from build123d import *

# Parameters (mm, degrees)
F1_DEPTH = 12.5
F2_W     = 25
F2_H     = 34
F3_DEPTH = 2.5
F4_W     = 25
F4_H     = 2
F5_DEPTH = 30
F6_W     = 2
F6_H     = 25
F7_DEPTH = 20
F8_W     = 32.5
F8_H     = 10
F9_DEPTH = 2


with BuildPart() as f1:
    # F0 (on Front) → F1 (new body, symmetric)
    with BuildSketch(Plane.XZ):
        Polygon((9.5, -9.5), (9.5, 9.5), (-9.5, 9.5), (-9.5, -9.5), (-5.75, -9.5), (-5.75, -6.75), (-6.75, -6.75), (-6.75, 6.75), (6.75, 6.75), (6.75, -6.75), (6.75, -9.5), align=None)
    extrude(amount=F1_DEPTH, both=True)

    # F2 (on face) → F3 (join)
    with BuildSketch(Plane(origin=(-9.5, 0, 0), x_dir=(0, -1, 0), z_dir=(-1, 0, 0))):
        with Locations((0, -7.5)):
            Rectangle(F2_W, F2_H)
    extrude(amount=-F3_DEPTH)

    # F4 (on face) → F5 (join)
    with BuildSketch(Plane(origin=(-9.5, 0, 0), x_dir=(0, -1, 0), z_dir=(-1, 0, 0))):
        with Locations((0, -23.5)):
            Rectangle(F4_W, F4_H)
    extrude(amount=F5_DEPTH)

    # F6 (on face) → F7 (join)
    with BuildSketch(Plane.XY.offset(-22.5)):
        with Locations((-38.5, 0)):
            Rectangle(F6_W, F6_H)
    extrude(amount=F7_DEPTH)

    # F8 (on face) → F9 (join)
    with BuildSketch(Plane.XZ.offset(12.5)):
        with Locations((-23.25, -19.5)):
            Rectangle(F8_W, F8_H)
    extrude(amount=-F9_DEPTH)


solid = f1.part
Verification items for the finished model (mm, model axes). A direction names the side the tool comes from. Round coordinates to 2 decimals unless told otherwise and drop trailing zeros. Write each loop counter-clockwise with the first axis right and the second up, starting at its lowest first coordinate (ties: lowest second). Pieces come first, ordered by that corner, then holes.
(1) Section check B-B (z = 3). Enter the section's corners in (x, y), plus the area to 4 significant figures.
Returned:
outline: (-9.5, -12.5) - (-6.75, -12.5) - (-6.75, 12.5) - (-9.5, 12.5) - close; (6.75, -12.5) - (9.5, -12.5) - (9.5, 12.5) - (6.75, 12.5) - close
area: 137.5 mm2
(2) Section check C-C (y = -9.25). Enter the section's corners in (x, z).
Returned:
outline: (-39.5, -24.5) - (-7, -24.5) - (-7, -9.5) - (-5.75, -9.5) - (-5.75, -6.75) - (-6.75, -6.75) - (-6.75, 6.75) - (6.75, 6.75) - (6.75, -9.5) - (9.5, -9.5) - (9.5, 9.5) - (-9.5, 9.5) - (-9.5, -22.5) - (-37.5, -22.5) - (-37.5, -2.5) - (-39.5, -2.5) - close
(3) Section check D-D (x = -35.5). Enter the section's corners in (y, z), plus the area to 3 significant figures.
Returned:
outline: (-12.5, -24.5) - (12.5, -24.5) - (12.5, -22.5) - (-10.5, -22.5) - (-10.5, -14.5) - (-12.5, -14.5) - close
area: 66.0 mm2
(4) Access from +Z, -Z, +X, -X, +Y, -Y to the whole of each face (thin tool, end or side, straight path). Record for faces 1 (the flat face through (-37.5, 0, -13)), 2 (the flat face through (8, 0, -9.5)), 3 (the flat face through (-6, 0, -6.75)), 4 (the flat face through (-24, -12, -14.5)).
Returned:
face 1: +Z, +Y
face 2: -Z, +X, +Y, -Y
face 3: +Y, -Y
face 4: +Z, +Y, -Y
(5) Mould release check, pull along X, two halves, no side actions. Record for faces 5 (the flat face through (0, 0, 6.75)), 6 (the flat face through (-7, 0, -17)), 7 (the flat face through (0, 0, 9.5)), 8 (the flat face through (-23, 1, -22.5)): pulls with the +X half, pulls with the -X half, needs draft (parallel to the pull), parting line crosses it, or undercut.
Returned:
face 5: undercut
face 6: pulls with the +X half
face 7: needs draft
face 8: undercut
(6) Material ranges on line 1 (X direction, y = 1.5, z = -12.5); line 2 (X direction, y = -9.25, z = -3); line 3 (X direction, y = 0.75, z = 5.5), recorded low to high.
Returned:
line 1: x = -39.5 to -37.5, -9.5 to -7
line 2: x = -39.5 to -37.5, -9.5 to -6.75, 6.75 to 9.5
line 3: x = -9.5 to -6.75, 6.75 to 9.5
(7) Section check A-A (z = -7.5). Enter the section's corners in (x, y).
Returned:
outline: (-39.5, -12.5) - (-37.5, -12.5) - (-37.5, 12.5) - (-39.5, 12.5) - close; (-9.5, -12.5) - (-5.75, -12.5) - (-5.75, 12.5) - (-9.5, 12.5) - close; (6.75, -12.5) - (9.5, -12.5) - (9.5, 12.5) - (6.75, 12.5) - close
(8) Depth check by flat-ended pin: pin 1 Ø12 at (y, z) = (5, -18) entering from +X; pin 2 Ø2 at (x, y) = (-38, -3.5) entering from +Z; pin 3 Ø5 at (y, z) = (6, 2) entering from -X. Enter the tip coordinate at first touch or a pass-through.
Returned:
pin 1: stops at x = -7
pin 2: stops at z = -2.5
pin 3: stops at x = -9.5
